Could you check a few things on this model? Use its own coordinates, in mm. A direction names the side the tool comes from. Give positions to 0.01 mm unless a question says otherwise; leave off trailing zeros. Order: outer loops, then holes, each group sorted by start corner. A loop starts at its lowest first (then second) coordinate and runs counter-clockwise, first axis right, second up. Notation, with made-up numbers: M 31.25,-23.75 L 73.25,-23.75 A20 cw 73.25,-8.75 Z; hole C 59.5,-14 d10. An arc over 180 degrees is marked long. Use a Markdown table: item, result. Add a question column.
Item 1: For faces 1 (the face through (2.375, 0, 0)), 2 (the face through (2, 0, -0.89)), 3 (the face through (-0.89, 0, -2)), 4 (the face through (-0.89, 0, 2)), 5 (the face through (2, 0, 0.89)), which set-ups out of +Z, -Z, +X, -X, +Y, -Y let a thin tool reach every point of the face, with its end or its side?
Item 2: Suppose I cut it at A-A on y = 1. Write out the boundary of the cut face in (x, z) (3 decimals), plus the area to 3 significant figures.
Item 3: Suppose I cut it at B-B on x = -1.7. Write out the boundary of the cut face in (y, z) (3 decimals), plus the area to 3 significant figures.
Item 4: I'm going to push flat-ended pins straight in: pin 1 Ø1.2 at (y, z) = (-7.5, 2) entering from -X; pin 2 Ø0.7 at (x, y) = (-2, -5.5) entering from +Z; pin 3 Ø1.2 at (y, z) = (0.5, 2) entering from +X. Where does each tip first touch, or does it pass through?
Item 5: If I drill on L1, parallel to X at y = 0.5, z = -1.5, over which ranges is the centre line in solid material (lowest first)? Write a range as from..to.
from build123d import *

# Parameters (mm, degrees)
F0_W     = 0.89
F0_H     = 0.89
F1_DEPTH = 15.705


with BuildPart() as f1:
    # F0 (on Front) → F1 (new body, symmetric)
    with BuildSketch(Plane.XZ):
        Polygon((-0.89, 0.89), (-2.375, 0.89), (-2.375, -0.89), (-0.89, -0.89), (-0.89, 0), align=None)
        Polygon((-0.89, 2.375), (-0.89, 0.89), (0, 0.89), (0.89, 0.89), (0.89, 2.375), align=None)
        with Locations((-0.445, 0.445)):
            Rectangle(F0_W, F0_H)
        with Locations((0.445, 0.445)):
            Rectangle(F0_W, F0_H)
        with Locations((-0.445, -0.445)):
            Rectangle(F0_W, F0_H)
        Polygon((0, -0.89), (-0.89, -0.89), (-0.89, -2.375), (0.89, -2.375), (0.89, -0.89), align=None)
        Polygon((2.375, 0.89), (0.89, 0.89), (0.89, 0), (0.89, -0.89), (2.375, -0.89), align=None)
        with Locations((0.445, -0.445)):
            Rectangle(F0_W, F0_H)
    extrude(amount=F1_DEPTH, both=True)


solid = f1.part
Findings below:
| question | item | result |
|---|---|---|
| 1 | face 1 | +Z, -Z, +X, +Y, -Y |
| 1 | face 2 | -Z, +X, +Y, -Y |
| 1 | face 3 | -Z, -X, +Y, -Y |
| 1 | face 4 | +Z, -X, +Y, -Y |
| 1 | face 5 | +Z, +X, +Y, -Y |
| 2 | outline | M -2.375,-0.89 L -0.89,-0.89 L -0.89,-2.375 L 0.89,-2.375 L 0.89,-0.89 L 2.375,-0.89 L 2.375,0.89 L 0.89,0.89 L 0.89,2.375 L -0.89,2.375 L -0.89,0.89 L -2.375,0.89 Z |
| 2 | area | 13.7 mm^2 |
| 3 | outline | M -15.705,-0.89 L 15.705,-0.89 L 15.705,0.89 L -15.705,0.89 Z |
| 3 | area | 55.9 mm^2 |
| 4 | pin 1 | stops at x = -0.89 |
| 4 | pin 2 | stops at z = 0.89 |
| 4 | pin 3 | stops at x = 0.89 |
| 5 | L1 | x = -0.89..0.89 |
